Read the model definition and answer for the solid it produces. Units are mm, in the model's axes. Face numbers are marked on the shaded views. Coordinates: 2 decimals unless noted, no trailing zeros. Order: outer loops, then holes, each group sorted by start corner. A loop starts at its lowest first (then second) coordinate and runs counter-clockwise, first axis right, second up. Notation, with made-up numbers: M 6.5,34.5 L 55.5,34.5 A30 ccw 55.5,56.5 Z; hole C 78.5,40 d11. An arc over 180 degrees is marked long. One line per question, with ' | ' between items. Start each with the question number.
1) Consider probe 1 along X at (y, z) = (0, 295); probe 2 along Z at (x, y) = (0, 30.1); probe 3 along Y at (x, z) = (-2, 242). Determine where each line is inside the solid, lowest interval first.
2) Find section B-B, the plane y = 0. Write down the section's boundary in (x, z).
3) Find section A-A, the plane x = -10. Write down the section's boundary in (y, z), plus the area to 3 significant figures.
4) The mould has two halves that part along X. Classify the marked faces 1 and 2: +X half, -X half, draft (parallel to the pull), parting line (faces both ways), or undercut.
5) Find section C-C, the plane z = 52. Write down the section's boundary in (x, y).
6) Given P1, Ø5, axis at x = 0, z = 408.41, coming from the +Y side; P2, Ø10, axis at x = -15, z = 160, coming from the +Y side; P3, Ø1, axis at x = 22, y = 23, coming from the -Z side; P4, Ø10, axis at x = 17.5, z = 149.5, coming from the -Y side, each flat-ended and moving along its own axis, determine where each tip first touches the part or whether it passes through.
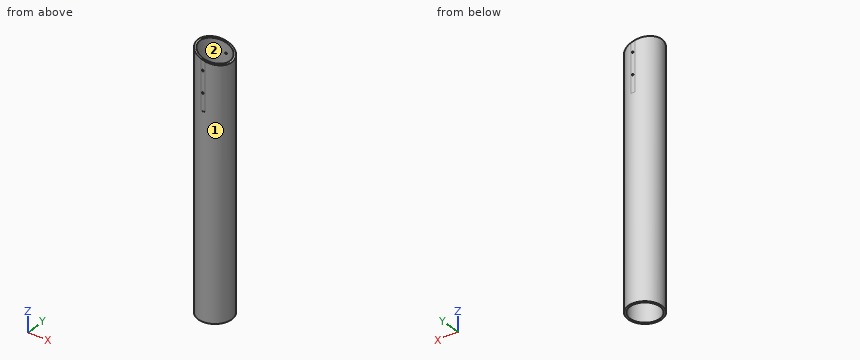
Autodesk Inventor part; units mm, degrees
ref_plane "Work Plane9" through (-31.5, 0, 476) normal (0.2588, 0, 0.9659) x (0, 1, 0)
ref_plane "Work Plane10" through (0, 31.5, 0) normal (0, 1, 0) x (-1, 0, 0)
ref_plane "Work Plane11" through (0, -31.5, 0) normal (0, -1, 0) x (1, 0, 0)
sketch "Sketch1" plane through (0, 0, 0) normal (0, 0, 1) x (1, 0, 0)
  circle A0 centre (0, 0) radius 31.5
  circle A1 centre (0, 0) radius 27.9
  dimension "d0" = 63
  dimension "d2" = 3.6
extrude "Extrusion1" add sketch "Sketch1" along normal blind 476
sketch "Sketch18" plane through (0, 0, 476) normal (0, 0, 1) x (1, 0, 0)
  circle A0 centre (0, 0) radius 27.9
  circle A1 centre (0, 0) radius 31.5
  point P0 (-31.5, 0)
ref_plane "Work Plane9" through (-31.5, 0, 476) normal (0.2588, 0, 0.9659) x (0, 1, 0)
sketch "Sketch19" plane through (-31.5, 0, 476) normal (0.2588, 0, 0.9659) x (0, 1, 0)
  line L0 (-31.6137, -94.9476) -> (64.4261, -94.9476)
  line L1 (64.4261, -94.9476) -> (64.4261, 6.6524)
  line L2 (64.4261, 6.6524) -> (-31.6137, 6.6524)
  line L3 (-31.6137, 6.6524) -> (-31.6137, -94.9476)
  point P0 (0, -153.6245)
  dimension "d61" = 101.6
extrude "Extrusion11" cut sketch "Sketch19" along normal blind 25.4
sketch "Sketch20" plane through (0, 0, 0) normal (0, 0, -1) x (-1, 0, 0)
  circle A0 centre (0, 0) radius 27.9
  circle A1 centre (0, 0) radius 31.5
  point P0 (0, 31.5)
  point P1 (0, -31.5)
ref_plane "Work Plane10" through (0, 31.5, 0) normal (0, 1, 0) x (-1, 0, 0)
ref_plane "Work Plane11" through (0, -31.5, 0) normal (0, -1, 0) x (1, 0, 0)
sketch "Sketch21" plane through (0, 31.5, 0) normal (0, 1, 0) x (-1, 0, 0)
  line L0 (-3.1444, 476) -> (6.8556, 476)
  line L1 (6.8556, 476) -> (6.8556, 376)
  line L2 (6.8556, 376) -> (-3.1444, 376)
  line L3 (-3.1444, 376) -> (-3.1444, 476)
  line L4 (1.8556, 476) -> (1.8556, 376) construction
  point P0 (0, 0)
  dimension "d64" = 10
  dimension "d65" = 100
  dimension "d82" = 376
extrude "flat1" cut sketch "Sketch21" against normal blind 0.254
sketch "Sketch22" plane through (0, -31.5, 0) normal (0, -1, 0) x (1, 0, 0)
  line L0 (-3.1568, 376) -> (6.8432, 376)
  line L1 (6.8432, 376) -> (6.8432, 476)
  line L2 (6.8432, 476) -> (-3.1568, 476)
  line L3 (-3.1568, 476) -> (-3.1568, 376)
  line L4 (1.8432, 476) -> (1.8432, 376) construction
  point P0 (0, 0)
  dimension "d68" = 10
  dimension "d69" = 100
  dimension "d83" = 376
extrude "flat2" cut sketch "Sketch22" against normal blind 0.254
sketch "Sketch23" plane through (0, -31.246, 0) normal (0, -1, 0) x (1, 0, 0)
  circle A0 centre (0, 448.4055) radius 1.4603
  circle A1 centre (0, 408.4055) radius 1.4603
  point P0 (-3.1568, 468.4055)
  point P1 (0, 0)
  dimension "d73" = 40
  dimension "d74" = 20
hole "Hole1" at (0, -31.246, 448.4055) at (0, -31.246, 408.4055) direction (0, 1, 0) diameter 3.175 end through all
properties part number "2r2scs" material "PVC-Piping"
Report:
1) probe 1: x = -31.5 to -27.9, 27.9 to 31.5 | probe 2: z = 0 to 406.82, 409.99 to 446.82, 449.99 to 467.56 | probe 3: y = -31.44 to -27.83, 27.83 to 31.44
2) outline: M -31.5,0 L -27.9,0 L -27.9,475.03 L -31.5,476 Z; M 27.9,0 L 31.5,0 L 31.5,459.12 L 27.9,460.08 Z
3) outline: M -29.87,0 L -26.05,0 L -26.05,470.24 L -29.87,470.24 Z; M 26.05,0 L 29.87,0 L 29.87,470.24 L 26.05,470.24 Z | area: 3,600 mm^2
4) face 1: parting line | face 2: undercut
5) outline: C 0,0 d63; hole C 0,0 d55.8
6) P1: stops at y = 31.25 | P2: stops at y = 29.87 | P3: stops at z = 0 | P4: stops at y = -28.91
